Work out the finished part from the listing and answer in its coordinate system (mm). Face numbers are marked on the shaded views. Round coordinates to 2 decimals unless told otherwise and drop trailing zeros. Order: outer loops, then holes, each group sorted by start corner. A loop starts at its lowest first (then second) coordinate and runs counter-clockwise, first axis right, second up. Notation, with made-up numbers: (37.5, 22.25) - (87.5, 22.25) arc R27 ccw to (87.5, 46.25) - close; hole circle Ø9 at (41.25, 76). An arc over 180 degrees is marked (long way). Use CSV: the item, a comma, the result in double quotes.
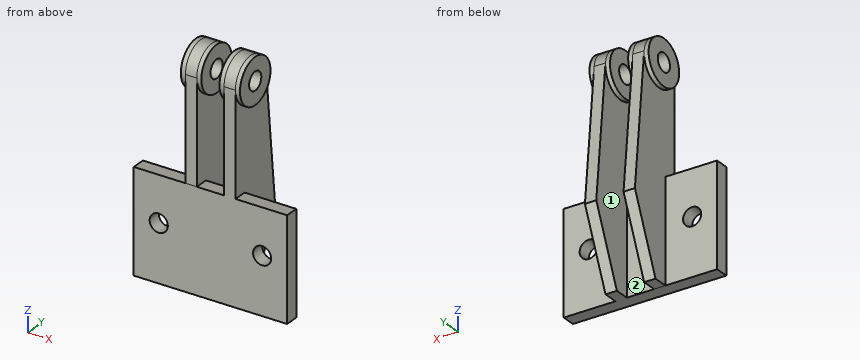
from build123d import *
from build123d.topology import SkipClean

# Parameters (mm, degrees)
SKETCH1_W           = 90
SKETCH1_H           = 12
BOSS_EXTRUDE1_DEPTH = 67.5
BOSS_EXTRUDE2_START = 12
BOSS_EXTRUDE2_DEPTH = 10
BOSS_EXTRUDE3_START = -14
SKETCH3_R           = 20
BOSS_EXTRUDE3_DEPTH = 18
HOLE1_D             = 16
HOLE2_D             = 16


with BuildPart() as part:
    # Sketch1 → Boss-Extrude1 (new, symmetric)
    with BuildSketch(Plane(origin=(0, 0, 0), x_dir=(0, 0, -1), z_dir=(1, 0, 0))):
        with Locations((45, 6)):
            Rectangle(SKETCH1_W, SKETCH1_H)
    extrude(amount=BOSS_EXTRUDE1_DEPTH, both=True)

    # Sketch2 → Boss-Extrude2 (add)
    with BuildSketch(Plane(origin=(0, 0, 0), x_dir=(0, 0, -1), z_dir=(1, 0, 0)).offset(BOSS_EXTRUDE2_START)):
        with BuildLine():
            Line((90, 12), (0, 12))
            Line((0, 12), (0, 0))
            Line((0, 0), (-90, 0))
            ThreePointArc((-90, 0), (-109.974333849, 18.987089694), (-92.023220861, 39.897401271))
            Line((-92.023220861, 39.897401271), (27, 52))
            Line((27, 52), (90, 25))
            Line((90, 25), (90, 12))
        make_face()
    boss_extrude2 = extrude(amount=BOSS_EXTRUDE2_DEPTH)

    # Sketch3 → Boss-Extrude3 (add)
    with SkipClean():  # the faces are left unmerged after this step: merging them gives an invalid solid
        with BuildSketch(Plane(origin=(22, 0, 0), x_dir=(0, 0, -1), z_dir=(1, 0, 0)).offset(BOSS_EXTRUDE3_START)):
            with Locations((-90, 20)):
                Circle(SKETCH3_R)
        boss_extrude3 = extrude(amount=BOSS_EXTRUDE3_DEPTH)

    # Mirror1: Boss-Extrude2, Boss-Extrude3 across plane
    with SkipClean():  # the faces are left unmerged after this step: merging them gives an invalid solid
        add(boss_extrude2.mirror(Plane(origin=(0, 0, 0), x_dir=(0, 0, 1), z_dir=(1, 0, 0))))
        add(boss_extrude3.mirror(Plane(origin=(0, 0, 0), x_dir=(0, 0, 1), z_dir=(1, 0, 0))))

    # Hole1 (through all)
    with Locations(Plane(origin=(26, 0, 0), x_dir=(0, 0, -1), z_dir=(1, 0, 0))):
        with Locations((-90, 20)):
            Hole(HOLE1_D / 2)

    # Hole2 (through all)
    with Locations(Plane(origin=(0, 12, 0), x_dir=(1, 0, 0), z_dir=(0, 1, 0))):
        with Locations((45.5, 40)):
            hole2 = Hole(HOLE2_D / 2)

    # Mirror2: Hole2 across plane
    with SkipClean():  # the faces are left unmerged after this step: merging them gives an invalid solid
        add(hole2.mirror(Plane(origin=(0, 0, 0), x_dir=(0, 0, 1), z_dir=(1, 0, 0))), mode=Mode.SUBTRACT)


solid = part.part
(1) Find section C-C (z = 45.5). Determine the outline of the cut face in (x, y), and give its area (3 significant figures).
Findings below:
outline,"(-22, 0) - (-12, 0) - (-12, 44.63) - (-22, 44.63) - close; (12, 0) - (22, 0) - (22, 44.63) - (12, 44.63) - close"
area,"893 mm²"
(2) Find section A-A (y = 20). Determine the outline of the cut face in (x, z).
Findings below:
outline,"(-26, 70) - (-22, 70) - (-22, -90) - (-12, -90) - (-12, 70) - (-8, 70) - (-8, 82) - (-26, 82) - close; (-26, 98) - (-8, 98) - (-8, 110) - (-26, 110) - close; (8, 70) - (12, 70) - (12, -90) - (22, -90) - (22, 70) - (26, 70) - (26, 82) - (8, 82) - close; (8, 98) - (26, 98) - (26, 110) - (8, 110) - close"
(3) Find section D-D (y = 4). Determine the outline of the cut face in (x, z).
Findings below:
outline,"(-67.5, -90) - (67.5, -90) - (67.5, 0) - (22, 0) - (22, 78) - (26, 78) - (26, 102) - (8, 102) - (8, 78) - (12, 78) - (12, 0) - (-12, 0) - (-12, 78) - (-8, 78) - (-8, 102) - (-26, 102) - (-26, 78) - (-22, 78) - (-22, 0) - (-67.5, 0) - close; hole circle Ø16 at (-45.5, -40); hole circle Ø16 at (45.5, -40)"
(4) Find the intervals of material crossed by L1, parallel to X at y = 19, z = 52.5; L2, parallel to Z at x = -45, y = 4; L3, parallel to Y at x = -38, z = -7, in increasing order. Write a range as from..to.
Findings below:
L1,"x = -22..-12, 12..22"
L2,"z = -90..-47.98, -32.02..0"
L3,"y = 0..12"
(5) Each of these flat-tipped pins is pushed along its axis until it touches: pin 1 (23 mm diameter, centred on x = 48, z = -57, fed in from +Y); pin 2 (3 mm diameter, centred on x = 10, y = 16, fed in from -Z); pin 3 (1.5 mm diameter, centred on x = -37, y = 11.5, fed in from +Z); pin 4 (8 mm diameter, centred on x = -37, z = -46, fed in from -Y). Where does it stop, or does it pass through?
Findings below:
pin 1,"stops at y = 12"
pin 2,"stops at z = 70.16"
pin 3,"stops at z = 0"
pin 4,"stops at y = 0"
(6) Find section B-B (x = 41). Determine the outline of the cut face in (y, z).
Findings below:
outline,"(0, -90) - (12, -90) - (12, -46.61) - (0, -46.61) - close; (0, -33.39) - (12, -33.39) - (12, 0) - (0, 0) - close"
(7) The mould has two halves that part along Z. Classify the marked faces 1 and 2: released by +Z, released by -Z, zero draft, split by the parting line, or undercut.
Findings below:
face 1,"undercut"
face 2,"zero draft"
